```python
from build123d import *

# Parameters (mm, degrees)
F0_R     = 8.45
F1_DEPTH = 5
F3_DEPTH = 5
F5_DEPTH = 9


# Not quite as in the source:
# - after a boolean that leaves OpenCascade's solid faulty, fix() repairs it
# - a feature names something its author has since deleted; it is built from what else it names


with BuildPart() as f1:
    # F0 (on Front) → F1 (new body)
    with BuildSketch(Plane.XZ):
        with BuildLine():
            ThreePointArc((14.975, 12.4899709767), (13.7885822331, 13.7885822331), (12.4899709767, 14.975))
            Line((12.4899709767, 14.975), (-12.4899709767, 14.975))
            ThreePointArc((-12.4899709767, 14.975), (-13.7885822331, 13.7885822331), (-14.975, 12.4899709767))
            Line((-14.975, 12.4899709767), (-14.975, -12.4899709767))
            ThreePointArc((-14.975, -12.4899709767), (-13.7885822331, -13.7885822331), (-12.4899709767, -14.975))
            Line((-12.4899709767, -14.975), (12.4899709767, -14.975))
            ThreePointArc((12.4899709767, -14.975), (13.7885822331, -13.7885822331), (14.975, -12.4899709767))
            Line((14.975, -12.4899709767), (14.975, 12.4899709767))
        make_face()
        Circle(F0_R, mode=Mode.SUBTRACT)
        with BuildLine():
            Line((-12.4899709767, 14.975), (12.4899709767, 14.975))
            ThreePointArc((12.4899709767, 14.975), (0, 19.5), (-12.4899709767, 14.975))
        make_face()
        with BuildLine():
            ThreePointArc((-12.4899709767, -14.975), (0, -19.5), (12.4899709767, -14.975))
            Line((12.4899709767, -14.975), (-12.4899709767, -14.975))
        make_face()
        with BuildLine():
            ThreePointArc((19.5, 0), (18.3338825675, 6.6421946674), (14.975, 12.4899709767))
            Line((14.975, 12.4899709767), (14.975, -12.4899709767))
            ThreePointArc((14.975, -12.4899709767), (18.3338825675, -6.6421946674), (19.5, 0))
        make_face()
        with BuildLine():
            Line((-14.975, -12.4899709767), (-14.975, 12.4899709767))
            ThreePointArc((-14.975, 12.4899709767), (-19.5, 0), (-14.975, -12.4899709767))
        make_face()
    extrude(amount=F1_DEPTH)

    # F2 (on face) → F3 (cut, through all)
    with BuildSketch(Plane(origin=(0, 0, 0), x_dir=(-1, 0, 0), z_dir=(0, 1, 0))):
        with BuildLine():
            ThreePointArc((12.4899709767, 14.975), (0, 19.5), (-12.4899709767, 14.975))
            Line((-12.4899709767, 14.975), (12.4899709767, 14.975))
        make_face()
        with BuildLine():
            Line((12.4899709767, -14.975), (-12.4899709767, -14.975))
            ThreePointArc((-12.4899709767, -14.975), (0, -19.5), (12.4899709767, -14.975))
        make_face()
    extrude(amount=-F3_DEPTH, mode=Mode.SUBTRACT)

    # F4 (on face) → F5 (join)
    with BuildSketch(Plane(origin=(0, 0, 0), x_dir=(-1, 0, 0), z_dir=(0, 1, 0))):
        with BuildLine():
            Line((-14.975, -12.4899709767), (-14.975, 12.4899709767))
            ThreePointArc((-14.975, 12.4899709767), (-19.5, 0), (-14.975, -12.4899709767))
        make_face()
        with BuildLine():
            ThreePointArc((14.975, -12.4899709767), (19.5, 0), (14.975, 12.4899709767))
            Line((14.975, 12.4899709767), (14.975, -12.4899709767))
        make_face()
    extrude(amount=F5_DEPTH)

    add(f1.part.fix(), mode=Mode.REPLACE)


solid = f1.part
```
Geometry check sheet. Reference: the model listing, model coordinates, mm. A direction names the side the tool comes from. Round coordinates to 2 decimals unless told otherwise and drop trailing zeros. Write each loop counter-clockwise with the first axis right and the second up, starting at its lowest first coordinate (ties: lowest second). Pieces come first, ordered by that corner, then holes. Notation, with made-up numbers: (5.5, 65) - (11.5, 65) arc R24 ccw to (11.5, 86) - close; hole circle Ø11 at (51.5, -36). An arc over 180 degrees is marked (long way). Write each question's results on one line, items separated by ' | '.
(1) Sectioned sample at A-A, the plane y = -2. Enter the section's corners in (x, z) (3 decimals), plus the area to 3 significant figures.
Computed:
outline: (-12.49, -14.975) - (12.49, -14.975) arc R19.5 ccw to (12.49, 14.975) - (-12.49, 14.975) arc R19.5 ccw to start; hole circle Ø16.9 at (0, 0) | area: 816 mm^2
(2) Depth check by flat-ended pin: pin 1 Ø1.5 at (y, z) = (0, -8) entering from -X; pin 2 Ø1.5 at (y, z) = (-1, -6) entering from -X; pin 3 Ø4.5 at (y, z) = (4.5, -4.5) entering from +X. Enter the tip coordinate at first touch or a pass-through.
Computed:
pin 1: stops at x = -18.1 | pin 2: stops at x = -18.78 | pin 3: stops at x = 19.37
(3) Draft check along Z on faces 3 (the face through (0, -2, 14.975)), 4 (the face through (0, -2, -14.975)), 5 (the face through (8.06, -2.46, 2.54)), 6 (the face through (-9, -5, 0)). Enter one of: pulls with the +Z half, pulls with the -Z half, needs draft (parallel to the pull), parting line crosses it, or undercut.
Computed:
face 3: pulls with the +Z half | face 4: pulls with the -Z half | face 5: undercut | face 6: needs draft
(4) Thickness scan on probe 1 along Z at (x, y) = (0, -3) (3 decimals); probe 2 along Y at (x, z) = (10.5, -4.25); probe 3 along X at (y, z) = (6.25, -6.75) (3 decimals). Record the ranges inside material, lowest first. Write a range as from..to.
Computed:
probe 1: z = -14.975..-8.45, 8.45..14.975 | probe 2: y = -5..0 | probe 3: x = -18.294..-14.975, 14.975..18.294
(5) Sectioned sample at D-D, the plane y = 5. Enter the section's corners in (x, z) (3 decimals).
Computed:
outline: (-14.975, -12.49) - (-14.975, 12.49) arc R19.5 ccw to start; (14.975, -12.49) arc R19.5 ccw to (14.975, 12.49) - close
(6) Sectioned sample at C-C, the plane z = 5. Enter the section's corners in (x, y) (3 decimals), plus the area to 3 significant figures.
Computed:
outline: (-18.848, -5) - (-6.812, -5) - (-6.812, 0) - (-14.975, 0) - (-14.975, 9) - (-18.848, 9) - close; (6.812, -5) - (18.848, -5) - (18.848, 9) - (14.975, 9) - (14.975, 0) - (6.812, 0) - close | area: 190 mm^2
(7) Set-up check for faces 1 (the face through (14.975, 4, 0)), 2 (the face through (17, 9, 0)): record each of +Z, -Z, +X, -X, +Y, -Y from which the full face is reachable in a straight line by a thin tool's end or side.
Computed:
face 1: +Z, -Z, +Y | face 2: +Z, -Z, +X, -X, +Y
(8) Sectioned sample at B-B, the plane x = 0. Enter the section's corners in (y, z) (3 decimals).
Computed:
outline: (-5, -14.975) - (0, -14.975) - (0, -8.45) - (-5, -8.45) - close; (-5, 8.45) - (0, 8.45) - (0, 14.975) - (-5, 14.975) - close
